Source: CAD feature listing. Evaluate the final solid. Frame: model axes, mm. A direction names the side the tool comes from. Coordinates: 2 decimals unless noted, no trailing zeros. Write each loop counter-clockwise with the first axis right and the second up, starting at its lowest first coordinate (ties: lowest second). Pieces come first, ordered by that corner, then holes. Notation, with made-up numbers: (11.25, 53) - (59.25, 53) arc R17 ccw to (59.25, 79) - close; hole circle Ø8 at (38.5, 18.25). An arc over 180 degrees is marked (long way). One line per question, with ' | ' between items. Start each with the question number.
Q1. Draft query along Z for faces 3 (the face through (-1.94, -31.23, 4.93)), 4 (the face through (-6.92, -15.13, 4.75)), 5 (the face through (2, -48, 20)), 6 (the face through (-5.72, -17.656, 5.978)). Return one class per face: +Z half, -Z half, draft (parallel to the pull), parting line (faces both ways), or undercut.
Q2. Cut plane D-D, the plane y = -46.5. Return loops of the section in (x, z), plus the area to 3 significant figures.
Q3. Line query: line 1 (X direction, y = -17, z = 5.5); line 2 (X direction, y = -43.67, z = 13); line 3 (Y direction, x = -0.5, z = 6.75). Output: solid intervals per line, ascending.
Q4. Contact query for flat-ended pins moving along their axis: P1, Ø5, axis at x = -6.5, z = 5.5, coming from the +Y side; P2, Ø8, axis at y = -37.5, z = 7, coming from the +X side; P3, Ø4, axis at x = -4.5, z = 12.5, coming from the -Y side. Output: stop coordinate, or through.
Q5. Cut plane B-B, the plane x = -2. Return loops of the section in (y, z), plus the area to 3 significant figures.
Q6. Access query for faces 1 (the face through (-1.9, -31.4, 0)), 2 (the face through (-3, -45, 10)). Directions: +Z, -Z, +X, -X, +Y, -Y. A direction counts if a zero-diameter tool reaches every point of the face in a straight line with its end or side. Return the directions, or none.
Q7. Cut plane A-A, the plane y = -29.67. Return loops of the section in (x, z), plus the area to 3 significant figures.
Q8. Cut plane C-C, the plane z = 3. Give the number of separate pieces and of enclosed holes in the cut face, plus the area to 3 significant figures.
Autodesk Inventor part; units mm, degrees
ref_plane "РабПлоскость1" through (0, 0, 0) normal (0, 0, 1) x (1, 0, 0)
ref_plane "РабПлоскость5" through (-9.7368, -21.67, 0) normal (-0.7071068, 0.7071068, 0) x (0, 0, 1)
ref_plane "YZ Plane" through (0, 0, 0) normal (1, 0, 0) x (0, 1, 0)
sketch "Эскиз1" plane through (0, 0, 0) normal (0, 0, 1) x (1, 0, 0)
  circle A0 centre (-1.7368, -21.67) radius 2.375
  circle A1 centre (-1.7368, -21.67) radius 7.5
  line L0 (-1.7368, -14.17) -> (-1.7368, -54.17) construction
  arc A2 (5.7632, -21.67) -> (-9.2368, -21.67) centre (-1.7368, -21.67) ccw
  circle A3 centre (-1.7368, -43.67) radius 9
  circle A4 centre (-1.7368, -43.67) radius 1.5
  circle A5 centre (-1.7368, -43.67) radius 5
  line L1 (-10.7368, -43.67) -> (-9.2368, -21.67)
  line L2 (7.2632, -43.67) -> (5.7632, -21.67)
  point P0 (0, 0)
  point P1 (-1.7368, -34.17)
  dimension "d1" = 15
  dimension "d3" = 18
  dimension "d4" = 3
  dimension "d9" = 10
  dimension "d36" = 22
extrude "Выдавливание1" add sketch "Эскиз1" along normal blind 20 contours L2 A3 L1 | A3 L2 | L1 A3
ref_plane "РабПлоскость1" through (0, 0, 0) normal (0, 0, 1) x (1, 0, 0)
sketch "Эскиз2" plane through (0, 0, 0) normal (0, 0, 1) x (1, 0, 0)
  arc A0 (-10.7011, -44.4704) -> (7.2269, -44.4779) centre (-1.7368, -43.67) ccw
  circle A1 centre (-1.7368, -46.2892) radius 1.5 construction
  line L0 (-1.7368, -46.2892) -> (-1.7368, -6.2497) construction
  line L1 (55.1846, -47.0725) -> (61.6072, -35.9345) construction
  line L2 (61.6072, -35.9345) -> (57.2758, -33.4368) construction
  line L3 (57.2758, -33.4368) -> (59.7378, -29.1672) construction
  line L4 (59.7378, -29.1672) -> (54.2369, -25.9951) construction
  line L5 (54.2369, -25.9951) -> (53.6124, -27.078) construction
  line L6 (53.6124, -27.078) -> (51.62, -25.929) construction
  line L7 (51.62, -25.929) -> (52.2444, -24.8462) construction
  line L8 (52.2444, -24.8462) -> (46.7434, -21.6741) construction
  line L9 (46.7434, -21.6741) -> (48.2421, -19.0752) construction
  line L10 (48.2421, -19.0752) -> (53.743, -22.2473) construction
  line L11 (53.743, -22.2473) -> (54.3674, -21.1644) construction
  line L12 (54.3674, -21.1644) -> (56.3599, -22.3134) construction
  line L13 (56.3599, -22.3134) -> (55.7355, -23.3962) construction
  line L14 (55.7355, -23.3962) -> (61.2364, -26.5683) construction
  line L15 (61.2364, -26.5683) -> (63.6984, -22.2987) construction
  line L16 (63.6984, -22.2987) -> (68.0299, -24.7964) construction
  line L17 (68.0299, -24.7964) -> (74.4526, -13.6584) construction
  line L18 (74.4526, -13.6584) -> (23.3414, 15.8145) construction
  arc A2 (23.3414, 15.8145) -> (19.2439, 14.7142) centre (21.8428, 13.2156) ccw construction
  line L19 (19.2439, 14.7142) -> (16.6854, 10.2772) construction
  arc A3 (12.8035, 9.064) -> (16.6854, 10.2772) centre (14.0865, 11.7758) ccw construction
  arc A4 (12.8035, 9.064) -> (-21.0534, -49.6498) centre (-1.7368, -21.67) ccw construction
  arc A5 (-20.1589, -53.6172) -> (-21.0534, -49.6498) centre (-22.7578, -52.1186) ccw construction
  line L20 (-20.1589, -53.6172) -> (-22.7175, -58.0542) construction
  arc A6 (-22.7175, -58.0542) -> (-21.6172, -62.1517) centre (-20.1186, -59.5528) ccw construction
  line L21 (-21.6172, -62.1517) -> (29.4939, -91.6246) construction
  line L22 (29.4939, -91.6246) -> (35.9166, -80.4866) construction
  line L23 (35.9166, -80.4866) -> (31.5851, -77.9889) construction
  line L24 (31.5851, -77.9889) -> (34.0472, -73.7193) construction
  line L25 (34.0472, -73.7193) -> (28.5462, -70.5472) construction
  line L26 (28.5462, -70.5472) -> (27.9218, -71.6301) construction
  line L27 (27.9218, -71.6301) -> (25.9293, -70.4811) construction
  line L28 (25.9293, -70.4811) -> (26.5537, -69.3983) construction
  line L29 (26.5537, -69.3983) -> (21.0528, -66.2262) construction
  line L30 (21.0528, -66.2262) -> (22.5514, -63.6273) construction
  line L31 (22.5514, -63.6273) -> (28.0524, -66.7994) construction
  line L32 (28.0524, -66.7994) -> (28.6768, -65.7165) construction
  line L33 (28.6768, -65.7165) -> (30.6693, -66.8655) construction
  line L34 (30.6693, -66.8655) -> (30.0448, -67.9483) construction
  line L35 (30.0448, -67.9483) -> (35.5458, -71.1204) construction
  line L36 (35.5458, -71.1204) -> (38.0078, -66.8508) construction
  line L37 (38.0078, -66.8508) -> (42.3393, -69.3485) construction
  line L38 (42.3393, -69.3485) -> (48.7619, -58.2105) construction
  line L39 (48.7619, -58.2105) -> (44.4305, -55.7128) construction
  line L40 (44.4305, -55.7128) -> (50.8531, -44.5748) construction
  line L41 (50.8531, -44.5748) -> (55.1846, -47.0725) construction
  circle A7 centre (-1.7368, -21.67) radius 2.375 construction
  circle A8 centre (-1.7368, -21.67) radius 5.5
  arc A9 (9.1272, -23.3947) -> (-12.5628, -23.6187) centre (-1.7368, -21.67) ccw
  line L42 (-12.7368, -21.67) -> (-10.7011, -44.4704)
  circle A10 centre (-1.7368, -43.67) radius 9 construction
  line L43 (9.2605, -21.9158) -> (7.2269, -44.4779)
  circle A11 centre (-1.7368, -43.67) radius 1.5
  circle A12 centre (-1.7368, -13.67) radius 1.575
  circle A13 centre (6.2632, -21.67) radius 1.575
  circle A14 centre (-1.7368, -29.67) radius 1.575
  circle A15 centre (-9.7368, -21.67) radius 1.575
  point P0 (0, 0)
  point P1 (-1.7368, -12.095)
  point P2 (-1.7368, -10.67)
  point P3 (-1.7368, -10.67)
  point P4 (7.8382, -21.67)
  point P5 (-1.7368, -31.245)
  point P6 (-11.3118, -21.67)
  dimension "d22" = 3.15
  dimension "d20" = 11
  dimension "d21" = 22
  dimension "d27" = 8
  dimension "d30" = 360
extrude "Выдавливание2" add sketch "Эскиз2" along normal blind 10 contours L42 A9 L43 A0
ref_plane "РабПлоскость5" through (-9.7368, -21.67, 0) normal (-0.7071068, 0.7071068, 0) x (0, 0, 1)
sketch "Эскиз4" plane through (-9.7368, -21.67, 0) normal (-0.7071068, 0.7071068, 0) x (0, 0, 1)
  line L0 (10, 1.575) -> (0, 1.575) construction
  line L1 (0, 9.7387) -> (10, 9.7387) construction
  line L2 (10, -3.8949) -> (0, -3.8949) construction
  line L3 (0, -3.8949) -> (0, -1.575) construction
  line L4 (0, -1.575) -> (10, -1.575) construction
  line L5 (10, -1.575) -> (10, -3.8949) construction
  line L6 (0, 15.0908) -> (10, 15.0908) construction
  line L7 (10, 15.0908) -> (10, 12.8887) construction
  line L8 (10, 12.8887) -> (0, 12.8887) construction
  line L9 (0, 12.8887) -> (0, 15.0908) construction
  line L10 (10, 1.575) -> (10, -1.575) construction
  line L11 (0, 12.8887) -> (0, 9.7387) construction
  circle A0 centre (6, 5.6568) radius 1.575
  line L12 (0, 1.575) -> (0, 9.7387)
  line L13 (10, 9.7387) -> (10, 1.575)
  point P0 (0, 22.208)
  dimension "d32" = 3.15
extrude "Выдавливание4" cut sketch "Эскиз4" along normal blind 10
properties part number "кривошип" material "Пластик САН"
Reply:
1) face 3: draft | face 4: undercut | face 5: +Z half | face 6: undercut
2) outline: (-10.28, 0) - (6.81, 0) - (6.81, 20) - (2.39, 20) - (2.39, 10) - (-5.86, 10) - (-5.86, 20) - (-10.28, 20) - close | area: 259 mm^2
3) line 1: x = -11.7 to -8.52, -5.06 to -4.64, 1.17 to 8.22 | line 2: x = -10.74 to -6.74, 3.26 to 7.26 | line 3: y = -52.58 to -44.52, -42.82 to -30.65, -28.69 to -27.03, -16.31 to -14.65, -12.69 to -10.74
4) P1: stops at y = -10.91 | P2: stops at x = 8.22 | P3: stops at y = -52.64
5) outline: (-52.67, 0) - (-45.15, 0) - (-45.15, 10) - (-48.66, 10) - (-48.66, 20) - (-52.67, 20) - close; (-42.19, 0) - (-31.22, 0) - (-31.22, 10) - (-34.67, 10) - (-34.67, 20) - (-38.68, 20) - (-38.68, 10) - (-42.19, 10) - close; (-28.12, 0) - (-27.16, 0) - (-27.16, 10) - (-28.12, 10) - close; (-16.18, 0) - (-15.22, 0) - (-15.22, 10) - (-16.18, 10) - close; (-12.12, 0) - (-10.67, 0) - (-10.67, 10) - (-12.12, 10) - close | area: 298 mm^2
6) face 1: -Z, +X, -X, +Y, -Y | face 2: +Z
7) outline: (-12.02, 0) - (-3.31, 0) - (-3.31, 10) - (-12.02, 10) - close; (-0.16, 0) - (8.56, 0) - (8.56, 10) - (-0.16, 10) - close | area: 174 mm^2
8) separate pieces: 1 | enclosed holes: 6 | area: 625 mm^2
